Read the model definition and answer for the solid it produces. Units are mm, in the model's axes. A direction names the side the tool comes from. Give positions to 0.01 mm unless a question says otherwise; leave off trailing zeros. Order: outer loops, then holes, each group sorted by start corner. A loop starts at its lowest first (then second) coordinate and runs counter-clockwise, first axis right, second up. Notation, with made-up numbers: (-14.75, 0) - (12.25, 0) arc R27 ccw to (12.25, 22) - close; hole circle Ø11 at (4.25, -15.75). An arc over 180 degrees is marked (long way). Write each question's results on one line, items separated by ' | '.
from build123d import *

# Parameters (mm, degrees)
SKETCH1_W           = 40
SKETCH1_H           = 20
BOSS_EXTRUDE1_DEPTH = 38
SKETCH2_R           = 1.5
CUT_EXTRUDE1_DEPTH  = 10
SKETCH3_W           = 20
SKETCH3_H           = 2
BOSS_EXTRUDE2_DEPTH = 9
SKETCH6_R           = 1.5
CUT_EXTRUDE2_DEPTH  = 41.82341542
SKETCH7_W           = 20
SKETCH7_H           = 2
BOSS_EXTRUDE5_DEPTH = 9
SKETCH8_R           = 1.504714294
CUT_EXTRUDE3_DEPTH  = 45.405116872
FILLET1_R           = 1


with BuildPart() as part:
    # Sketch1 → Boss-Extrude1 (new body)
    with BuildSketch(Plane(origin=(0, 0, 0), x_dir=(1, 0, 0), z_dir=(0, 1, 0))):
        with Locations((-2.631578947, -3.684210526)):
            Rectangle(SKETCH1_W, SKETCH1_H)
    extrude(amount=BOSS_EXTRUDE1_DEPTH)

    # Sketch2 → Cut-Extrude1 (cut)
    with BuildSketch(Plane(origin=(0, 38, 0), x_dir=(1, 0, 0), z_dir=(0, 1, 0))):
        with Locations(Location((7.368421053, -3.684210526, 0), (0, 0, 270))):
            Circle(SKETCH2_R)
    extrude(amount=-CUT_EXTRUDE1_DEPTH, mode=Mode.SUBTRACT)

    # Sketch3 → Boss-Extrude2 (add)
    with BuildSketch(Plane(origin=(17.368421053, 0, 0), x_dir=(0, 0, -1), z_dir=(1, 0, 0))):
        with Locations((-3.684210526, 27)):
            Rectangle(SKETCH3_W, SKETCH3_H)
    extrude(amount=BOSS_EXTRUDE2_DEPTH)

    # Sketch6 → Cut-Extrude2 (cut, through all)
    with BuildSketch(Plane(origin=(0, 28, 0), x_dir=(1, 0, 0), z_dir=(0, 1, 0))):
        with Locations(Location((22.368421053, 1.315789474, 0), (0, 0, 270))):
            Circle(SKETCH6_R)
        with Locations(Location((22.368421053, -8.684210526, 0), (0, 0, 270))):
            Circle(SKETCH6_R)
    extrude(amount=-CUT_EXTRUDE2_DEPTH, mode=Mode.SUBTRACT)

    # Sketch7 → Boss-Extrude5 (add)
    with BuildSketch(Plane.ZY.offset(22.631578947)):
        with Locations((3.684210526, 27)):
            Rectangle(SKETCH7_W, SKETCH7_H)
    extrude(amount=BOSS_EXTRUDE5_DEPTH)

    # Sketch8 → Cut-Extrude3 (cut, through all)
    with BuildSketch(Plane(origin=(0, 28, 0), x_dir=(1, 0, 0), z_dir=(0, 1, 0))):
        with Locations(Location((-27.631578947, 1.315789474, 0), (0, 0, 270))):
            Circle(SKETCH8_R)
        with Locations(Location((-27.631578947, -8.684210526, 0), (0, 0, 270))):
            Circle(SKETCH8_R)
    extrude(amount=-CUT_EXTRUDE3_DEPTH, mode=Mode.SUBTRACT)

    # Fillet1
    fillet1_edges = [part.edges().sort_by_distance(p)[0] for p in [
        (17.368421053, 38, 3.684210526),
        (-2.631578947, 38, -6.315789474),
        (17.368421053, 26, 3.684210526),
        (26.368421053, 27, 13.684210526),
        (26.368421053, 27, -6.315789474),
        (17.368421053, 28, 3.684210526),
        (-22.631578947, 38, 3.684210526),
        (-2.631578947, 0, -6.315789474),
        (17.368421053, 0, 3.684210526),
        (-22.631578947, 26, 3.684210526),
        (-31.631578947, 27, -6.315789474),
        (-31.631578947, 27, 13.684210526),
        (-22.631578947, 28, 3.684210526),
        (-2.631578947, 0, 13.684210526),
        (-22.631578947, 0, 3.684210526),
        (-2.631578947, 38, 13.684210526),
    ]]
    fillet(fillet1_edges, radius=FILLET1_R)


solid = part.part
(1) For faces 4 (the face through (22, 26, 4)), 5 (the face through (-28, 26, 4)), 6 (the face through (8.382, 33.07, 2.579)), determine the directions among +Z, -Z, +X, -X, +Y, -Y from which every point of the face is accessible in a straight line to the end or side of a thin tool.
Conclusion:
face 4: +Z, -Z, +X, -Y | face 5: +Z, -Z, -X, -Y | face 6: +Y
(2) Section C-C (x = 20) is taken. Give the vertices of the cut face in (y, z), plus the area to 3 significant figures.
Conclusion:
outline: (26, -6.32) - (28, -6.32) - (28, 13.68) - (26, 13.68) - close | area: 40.0 mm^2
(3) Section D-D (y = 13) is taken. Give the vertices of the cut face in (x, z).
Conclusion:
outline: (-22.63, -6.32) - (17.37, -6.32) - (17.37, 13.68) - (-22.63, 13.68) - close
(4) Section A-A (z = 1.25) is taken. Give the vertices of the cut face in (x, y).
Conclusion:
outline: (-31.63, 26) - (-23.63, 26) arc R1 cw to (-22.63, 25) - (-22.63, 1) arc R1 ccw to (-21.63, 0) - (16.37, 0) arc R1 ccw to (17.37, 1) - (17.37, 25) arc R1 cw to (18.37, 26) - (26.37, 26) - (26.37, 28) - (18.37, 28) arc R1 cw to (17.37, 29) - (17.37, 37) arc R1 ccw to (16.37, 38) - (-21.63, 38) arc R1 ccw to (-22.63, 37) - (-22.63, 29) arc R1 cw to (-23.63, 28) - (-31.63, 28) - close
(5) Each of these flat-tipped pins is pushed along its axis until it touches: pin 1 (3 mm diameter, centred on y = 31, z = 3.5, fed in from +X); pin 2 (6.5 mm diameter, centred on x = -27.5, z = 2.5, fed in from -Y); pin 3 (6.5 mm diameter, centred on x = 21, z = 1.5, fed in from +Y). Where does it stop, or does it pass through?
Conclusion:
pin 1: x = 17.37 | pin 2: y = 26 | pin 3: y = 28.21
(6) The mould has two halves that part along X. Classify faces 1 (the face through (7, 28, 4)), 2 (the face through (-31.632, 27, 4)), 3 (the face through (-28, 28, 4)): pulls with the +X half, pulls with the -X half, needs draft (parallel to the pull), parting line crosses it, or undercut.
Conclusion:
face 1: undercut | face 2: pulls with the -X half | face 3: needs draft
(7) Section B-B (y = 34) is taken. Give the vertices of the cut face in (x, z), plus the area to 3 significant figures.
Conclusion:
outline: (-22.63, -6.32) - (17.37, -6.32) - (17.37, 13.68) - (-22.63, 13.68) - close; hole circle Ø3 at (7.37, 3.68) | area: 793 mm^2
(8) Consider probe 1 along X at (y, z) = (9, 7.5); probe 2 along Y at (x, z) = (19, 12.5); probe 3 along X at (y, z) = (31, 3). Determine where each line is inside the solid, lowest interval first. Write a range as [from, to].
Conclusion:
probe 1: [-22.63, 17.37] | probe 2: [26, 28] | probe 3: [-22.63, 6.03], [8.7, 17.37]
